For this review, take the finished solid that the model builds, in its own axes (mm). Face numbers are marked on the shaded views. A direction names the side the tool comes from. Give positions to 0.01 mm unless a question says otherwise; leave off trailing zeros. Loops run counter-clockwise (first coordinate to the right, second up) from the corner with the lowest first, then second, coordinate; pieces in that order, holes last. Notation, with made-up numbers: (39, 47) - (63, 47) arc R16 ccw to (63, 73) - close; hole circle Ø8 at (80.5, -27.75). An arc over 180 degrees is marked (long way). Answer in a Markdown table with one row per item.
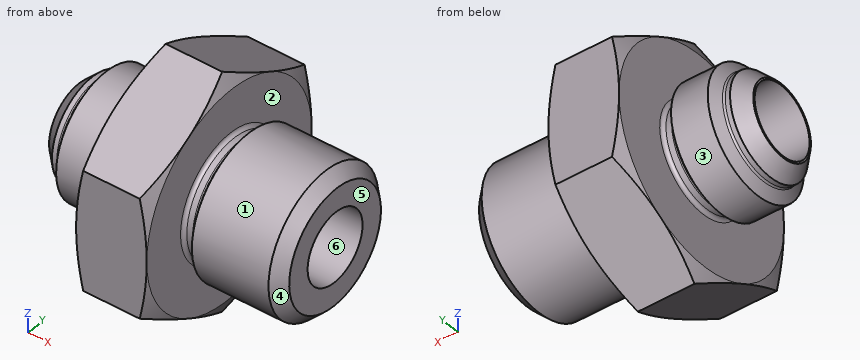
```python
from build123d import *

# Parameters (mm, degrees)
CUT_EXTRUDE1_START = -21
CUT_EXTRUDE1_DEPTH = 31.137402936
CIRPATTERN1_COUNT  = 6


with BuildPart() as part:
    # Sketch1 → Revolve1 (revolve)
    with BuildSketch(Plane(origin=(0, 0, 0), x_dir=(1, 0, 0), z_dir=(0, 1, 0))):
        with BuildLine():
            Line((6.500562053, 7.08), (6.500562053, 12))
            Line((6.500562053, 12), (3.500562053, 19))
            Line((3.500562053, 19), (1.500562053, 19))
            Line((1.500562053, 19), (-1.499437947, 12))
            Line((-1.499437947, 12), (-1.499437947, 6.08031838))
            ThreePointArc((-1.499437947, 6.08031838), (-1.616595234, 5.797475668), (-1.899437947, 5.68031838))
            Line((-1.899437947, 5.68031838), (-2.544567646, 5.68031838))
            ThreePointArc((-2.544567646, 5.68031838), (-2.670163765, 5.700547903), (-2.783056135, 5.759190305))
            Line((-2.783056135, 5.759190305), (-3.499437947, 7))
            Line((-3.499437947, 7), (-7.656522503, 7))
            Line((-7.656522503, 7), (-8.366963495, 5.769480105))
            ThreePointArc((-8.366963495, 5.769480105), (-8.485178679, 5.703267117), (-8.618716483, 5.68031838))
            Line((-8.618716483, 5.68031838), (-9.156522503, 5.68031838))
            Line((-9.156522503, 5.68031838), (-10.636840883, 4.2))
            Line((-10.636840883, 4.2), (-10.636840883, 4))
            Line((-10.636840883, 4), (18.500562053, 4))
            Line((18.500562053, 4), (18.500562053, 6.68))
            Line((18.500562053, 6.68), (17.180562053, 8))
            Line((17.180562053, 8), (8.500562053, 8))
            Line((8.500562053, 8), (7.945301013, 7.038259666))
            ThreePointArc((7.945301013, 7.038259666), (7.81516358, 6.782765973), (7.547484793, 6.68))
            Line((7.547484793, 6.68), (6.900562053, 6.68))
            ThreePointArc((6.900562053, 6.68), (6.617719341, 6.797157288), (6.500562053, 7.08))
        make_face()
    revolve(axis=Axis((-84.410714624, 0, 0), (1, 0, 0)))

    # Sketch2 → Cut-Extrude1 (cut)
    with BuildSketch(Plane.ZY.offset(1.499437947).offset(CUT_EXTRUDE1_START)):
        Polygon((-116.355697184, 12), (-14.730919863, 12), (14.730919863, 12), (116.355697184, 12), (116.355697184, 215.249554642), (-116.355697184, 215.249554642), align=None)
    cut_extrude1 = extrude(amount=CUT_EXTRUDE1_DEPTH, mode=Mode.SUBTRACT)

    # CirPattern1: Cut-Extrude1 ×6 about axis
    cirpattern1_axis = Axis((-84.410714624, 0, 0), (1, 0, 0))
    for i in range(1, CIRPATTERN1_COUNT):
        add(cut_extrude1.rotate(cirpattern1_axis, i * 360 / CIRPATTERN1_COUNT), mode=Mode.SUBTRACT)


solid = part.part
```
1. For the marked faces 1, 2 and 3, list the 3-axis set-ups (+Z, -Z, +X, -X, +Y, -Y) from which the entire face can be reached by the end or side of a thin tool; tool diameter is ignored.
Values:
| item | result |
|---|---|
| face 1 | +X |
| face 2 | none |
| face 3 | -X |
2. Mouldability with a two-part tool opening along Y and no side actions: class the marked faces 4, 5 and 6 as released by +Y, released by -Y, zero draft, split by the parting line, or undercut.
Values:
| item | result |
|---|---|
| face 4 | split by the parting line |
| face 5 | zero draft |
| face 6 | undercut |
3. We need section C-C, the plane x = 15.75. Give the boundary of the cut face in (y, z).
Values:
| item | result |
|---|---|
| outline | circle Ø16 at (0, 0); hole circle Ø8 at (0, 0) |
4. We need section A-A, the plane x = 1.5. Give the boundary of the cut face in (y, z).
Values:
| item | result |
|---|---|
| outline | (-12, -6.93) - (0, -13.86) - (12, -6.93) - (12, 6.93) - (0, 13.86) - (-12, 6.93) - close; hole circle Ø8 at (0, 0) |
5. Clearance check with flat-ended pins moving along their axes: pin 1 (1 mm diameter, centred on x = 1, y = 1, fed in from -Z); pin 2 (10 mm diameter, centred on y = 2, z = 9.5, fed in from -X); pin 3 (1.5 mm diameter, centred on x = 10, z = -7, fed in from +Y); pin 4 (6.5 mm diameter, centred on y = 0, z = 0, fed in from +X). State where each tip first meets the part, or that it passes through.
Values:
| item | result |
|---|---|
| pin 1 | stops at z = -13.57 |
| pin 2 | stops at x = -10.13 |
| pin 3 | stops at y = 4.99 |
| pin 4 | passes through |
6. We need section B-B, the plane x = -5. Give the boundary of the cut face in (y, z).
Values:
| item | result |
|---|---|
| outline | circle Ø14 at (0, 0); hole circle Ø8 at (0, 0) |
7. Wall thickness on line 1 (Y direction, x = 9.75, z = 0); line 2 (X direction, y = 0, z = -10.5); line 3 (Y direction, x = 12.5, z = 2.5): over which ranges is each line inside the solid? List them lowest first. Write a range as [from, to].
Values:
| item | result |
|---|---|
| line 1 | y = [-8, -4], [4, 8] |
| line 2 | x = [-1.5, 6.5] |
| line 3 | y = [-7.6, -3.12], [3.12, 7.6] |
